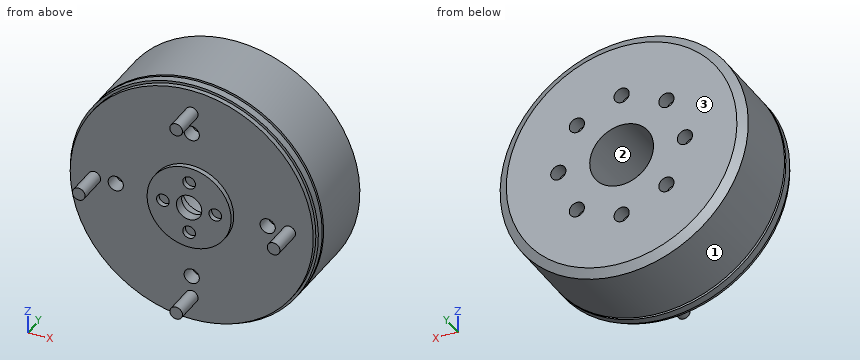
```python
from build123d import *

# Parameters (mm, degrees)
SKETCH_1_R               = 24.5
EXTRUDE_1_DEPTH          = 17
SKETCH_3_W               = 2.337455655
SKETCH_3_H               = 0.503987985
CHAMFER_1_SIZE           = 1
CHAMFER_1_SIZE2          = 1.732050808
SKETCH_4_R               = 24
EXTRUDE_2_DEPTH          = 1
SKETCH_5_R               = 8.3
EXTRUDE_3_DEPTH          = 1
SKETCH_6_R               = 6.3
CUT_EXTRUDE_1_DEPTH      = 14
SKETCH_7_R               = 4
CUT_EXTRUDE_2_DEPTH      = 3
SKETCH_8_R               = 2.5
CUT_EXTRUDE_3_DEPTH      = 2
SKETCH_9_R               = 1.5
CUT_EXTRUDE_4_DEPTH      = 3
PATTERN_CIRCULAR_1_COUNT = 8
SKETCH_12_R              = 1.5
CUT_EXTRUDE_5_DEPTH      = 3
PATTERN_CIRCULAR_2_COUNT = 4
SKETCH_15_R              = 1.25
CUT_EXTRUDE_8_DEPTH      = 1
PATTERN_CIRCULAR_4_COUNT = 4
SKETCH_16_R              = 1.25
EXTRUDE_4_DEPTH          = 6
PATTERN_CIRCULAR_5_COUNT = 4


with BuildPart() as part:
    # 草图1 → 凸台-拉伸1 (new body)
    with BuildSketch(Plane(origin=(0, 0, 0), x_dir=(1, 0, 0), z_dir=(0, 1, 0))):
        with Locations(Location((0, 0, 0), (0, 0, 270))):
            Circle(SKETCH_1_R)
    extrude(amount=EXTRUDE_1_DEPTH)

    # 草图3 → 切除-旋转1 (revolve, cut)
    with BuildSketch(Plane(origin=(0, 0, 0), x_dir=(0, 0, -1), z_dir=(1, 0, 0)), mode=Mode.PRIVATE) as cut_revolve_1_sk:
        with Locations((-24.668727827, 1.751993993)):
            Rectangle(SKETCH_3_W, SKETCH_3_H)
    revolve(cut_revolve_1_sk.sketch.rotate(Axis((0, 0, 0), (0, 1, 0)), 180), axis=Axis((0, 0, 0), (0, 1, 0)), mode=Mode.SUBTRACT)

    # 倒角1
    chamfer_1_edges = [part.edges().sort_by_distance(p)[0] for p in [
        (0, 17, -24.5),
    ]]
    chamfer_1_side = [part.faces().sort_by_distance(p)[0] for p in [
        (0, 9.501993992, -24.5),
    ]]
    chamfer(chamfer_1_edges, length=CHAMFER_1_SIZE, length2=CHAMFER_1_SIZE2, reference=chamfer_1_side[0])

    # 草图4 → 凸台-拉伸2 (add)
    with BuildSketch(Plane.XZ):
        with Locations(Location((0, 0, 0), (0, 0, 270))):
            Circle(SKETCH_4_R)
    extrude(amount=EXTRUDE_2_DEPTH)

    # 草图5 → 凸台-拉伸3 (add)
    with BuildSketch(Plane.XZ.offset(1)):
        with Locations(Location((0, 0, 0), (0, 0, 270))):
            Circle(SKETCH_5_R)
    extrude(amount=EXTRUDE_3_DEPTH)

    # 草图6 → 切除-拉伸1 (cut)
    with BuildSketch(Plane(origin=(0, 17, 0), x_dir=(1, 0, 0), z_dir=(0, 1, 0))):
        with Locations(Location((0, 0, 0), (0, 0, 270))):
            Circle(SKETCH_6_R)
    extrude(amount=-CUT_EXTRUDE_1_DEPTH, mode=Mode.SUBTRACT)

    # 草图7 → 切除-拉伸2 (cut)
    with BuildSketch(Plane(origin=(0, 3, 0), x_dir=(1, 0, 0), z_dir=(0, 1, 0))):
        with Locations(Location((0, 0, 0), (0, 0, 270))):
            Circle(SKETCH_7_R)
    extrude(amount=-CUT_EXTRUDE_2_DEPTH, mode=Mode.SUBTRACT)

    # 草图8 → 切除-拉伸3 (cut)
    with BuildSketch(Plane(origin=(0, 0, 0), x_dir=(1, 0, 0), z_dir=(0, 1, 0))):
        with Locations(Location((0, 0, 0), (0, 0, 270))):
            Circle(SKETCH_8_R)
    extrude(amount=-CUT_EXTRUDE_3_DEPTH, mode=Mode.SUBTRACT)

    # 草图9 → 切除-拉伸4 (cut)
    with BuildSketch(Plane(origin=(0, 17, 0), x_dir=(1, 0, 0), z_dir=(0, 1, 0))):
        with Locations(Location((0, 12.5, 0), (0, 0, 270))):
            Circle(SKETCH_9_R)
    cut_extrude_4 = extrude(amount=-CUT_EXTRUDE_4_DEPTH, mode=Mode.SUBTRACT)

    # 阵列(圆周)1: 切除-拉伸4 ×8 about axis
    pattern_circular_1_axis = Axis((0, 0, 0), (0, 1, 0))
    for i in range(1, PATTERN_CIRCULAR_1_COUNT):
        add(cut_extrude_4.rotate(pattern_circular_1_axis, i * 360 / PATTERN_CIRCULAR_1_COUNT), mode=Mode.SUBTRACT)

    # 草图12 → 切除-拉伸5 (cut)
    with BuildSketch(Plane.XZ.offset(1)):
        with Locations(Location((0, 15, 0), (0, 0, 270))):
            Circle(SKETCH_12_R)
    cut_extrude_5 = extrude(amount=-CUT_EXTRUDE_5_DEPTH, mode=Mode.SUBTRACT)

    # 阵列(圆周)2: 切除-拉伸5 ×4 about axis
    pattern_circular_2_axis = Axis((0, 0, 0), (0, 1, 0))
    for i in range(1, PATTERN_CIRCULAR_2_COUNT):
        add(cut_extrude_5.rotate(pattern_circular_2_axis, i * 360 / PATTERN_CIRCULAR_2_COUNT), mode=Mode.SUBTRACT)

    # 草图15 → 切除-拉伸8 (cut)
    with BuildSketch(Plane.XZ.offset(2)):
        with Locations(Location((0, 5.172485404, 0), (0, 0, 270))):
            Circle(SKETCH_15_R)
    cut_extrude_8 = extrude(amount=-CUT_EXTRUDE_8_DEPTH, mode=Mode.SUBTRACT)

    # 阵列(圆周)4: 切除-拉伸8 ×4 about axis
    pattern_circular_4_axis = Axis((0, 0, 0), (0, 1, 0))
    for i in range(1, PATTERN_CIRCULAR_4_COUNT):
        add(cut_extrude_8.rotate(pattern_circular_4_axis, i * 360 / PATTERN_CIRCULAR_4_COUNT), mode=Mode.SUBTRACT)

    # 草图16 → 凸台-拉伸4 (add)
    with BuildSketch(Plane.XZ.offset(1)):
        with Locations(Location((0, 19.25, 0), (0, 0, 270))):
            Circle(SKETCH_16_R)
    extrude_4 = extrude(amount=EXTRUDE_4_DEPTH)

    # 阵列(圆周)5: 凸台-拉伸4 ×4 about axis
    pattern_circular_5_axis = Axis((0, 0, 0), (0, 1, 0))
    for i in range(1, PATTERN_CIRCULAR_5_COUNT):
        add(extrude_4.rotate(pattern_circular_5_axis, i * 360 / PATTERN_CIRCULAR_5_COUNT))


solid = part.part
```
The model under review builds one solid part; all positions refer to its coordinate system, in mm. Face numbers are marked on the shaded views. Round coordinates to 2 decimals unless told otherwise and drop trailing zeros. Write each loop counter-clockwise with the first axis right and the second up, starting at its lowest first coordinate (ties: lowest second). Pieces come first, ordered by that corner, then holes. Notation, with made-up numbers: (7.5, -26.75) - (24.5, -26.75) arc R26 cw to (24.5, 11.25) - close; hole circle Ø11 at (5, -15.5). An arc over 180 degrees is marked (long way). One line per question, with ' | ' between items.
Item 1: The part is to be moulded in two halves that separate along Z. For the marked faces 1, 2 and 3, say which applies: pulls with the +Z half, pulls with the -Z half, needs draft (parallel to the pull), parting line crosses it, or undercut.
Resolved:
face 1: parting line crosses it | face 2: undercut | face 3: needs draft
Item 2: Add section A-A, the plane y = 8. Give the boundary of the cut face in (x, z).
Resolved:
outline: circle Ø49 at (0, 0); hole circle Ø12.6 at (0, 0)
Item 3: To check wall thickness, follow probe 1 along Z at (x, y) = (9, 16.25); probe 2 along Y at (x, z) = (19, 12.5); probe 3 along Y at (x, z) = (1, -3). State the ranges of each line that lie inside material, in increasing order.
Resolved:
probe 1: z = -22.32 to -10.33, -7.35 to 7.35, 10.33 to 22.32 | probe 2: y = -1 to 17 | probe 3: y = -2 to 0
Item 4: For P1, Ø3, axis at y = 8, z = -11.5, coming from the -X side; P2, Ø2, axis at x = 5.17, z = 0, coming from the +Y side; P3, Ø7.5, axis at x = 0, z = 0, coming from the +Y side, all flat-tipped, find the tip position at first contact; note any pin that passes through.
Resolved:
P1: stops at x = -22.37 | P2: stops at y = 3 | P3: stops at y = 0
